Part model, mm, in its own coordinate system. A direction names the side the tool comes from. Round coordinates to 2 decimals unless told otherwise and drop trailing zeros. Write each loop counter-clockwise with the first axis right and the second up, starting at its lowest first coordinate (ties: lowest second). Pieces come first, ordered by that corner, then holes. Notation, with made-up numbers: M 41,19 L 58,19 A20 cw 58,43 Z; hole C -2.75,-4.75 d6. An arc over 180 degrees is marked long. One line per question, with ' | ' between items. Start each with the question number.
1) Saw through at C-C (z = 0). List the corners of the cut face in (x, y) (3 decimals).
2) Saw through at B-B (y = -8.75). List the corners of the cut face in (x, z) (3 decimals).
3) Saw through at A-A (x = 0). List the corners of the cut face in (y, z) (3 decimals), plus the area to 3 significant figures.
4) Drop flat-ended pins along their axis: pin 1 Ø0.5 at (x, y) = (11, -5) entering from -Z; pin 2 Ø3 at (y, z) = (-17.5, -0.5) entering from -X; pin 3 Ø4 at (y, z) = (-7.5, 5) entering from -X (3 decimals); pin 4 Ø1.5 at (x, y) = (-7, -18) entering from -Z. Give the stop position or say it passes through.
5) Saw through at D-D (y = -15.25). List the corners of the cut face in (x, z).
6) Tool access for faces 1 (the face through (-11, -5, 2.35)), 2 (the face through (-11, -5, -2.35)), 3 (the face through (10.325, -5, -5)): list every direction of +Z, -Z, +X, -X, +Y, -Y with a clear straight run to the whole face (end or side of a thin tool).
7) Wall check: probe 1 along Y at (x, z) = (11.75, 2); probe 2 along X at (y, z) = (-1.5, -5.75) (3 decimals); probe 3 along Y at (x, z) = (-2.5, 6.25). Give the ranges that are in metal, low to high. Write a range as [from, to].
```python
from build123d import *

# Parameters (mm, degrees)
F1_DEPTH = 10.2
F2_R     = 2
F3_R     = 7.65
F4_DEPTH = 6.8
F5_SIZE  = 3
F6_R     = 5.9
F7_DEPTH = 5


with BuildPart() as f1:
    # F0 (on Front) → F1 (new body)
    with BuildSketch(Plane.XZ):
        Polygon((10.325, 2.35), (10.325, 10.375), (-10.325, 10.375), (-10.325, 2.35), (-13.325, 2.35), (-13.325, -2.35), (-10.325, -2.35), (-10.325, -10.375), (10.325, -10.375), (10.325, -2.35), (13.325, -2.35), (13.325, 2.35), align=None)
    extrude(amount=F1_DEPTH)

    # F2
    f2_edges = [f1.edges().sort_by_distance(p)[0] for p in [
        (-13.325, -5.1, -2.35),
        (-13.325, -5.1, 2.35),
        (13.325, -5.1, -2.35),
        (13.325, -5.1, 2.35),
    ]]
    fillet(f2_edges, radius=F2_R)

    # F3 (on face) → F4 (join)
    with BuildSketch(Plane.XZ.offset(10.2)):
        Circle(F3_R)
    extrude(amount=F4_DEPTH)

    # F5
    f5_edges = [f1.edges().sort_by_distance(p)[0] for p in [
        (-10.325, -5.1, -10.375),
        (-10.325, -5.1, 10.375),
        (10.325, -5.1, -10.375),
        (10.325, -5.1, 10.375),
    ]]
    chamfer(f5_edges, length=F5_SIZE)

    # F6 (on face) → F7 (join)
    with BuildSketch(Plane.XZ.offset(17)):
        Circle(F6_R)
    extrude(amount=F7_DEPTH)


solid = f1.part
```
Answer key:
1) outline: M -13.325,-10.2 L -7.65,-10.2 L -7.65,-17 L -5.9,-17 L -5.9,-22 L 5.9,-22 L 5.9,-17 L 7.65,-17 L 7.65,-10.2 L 13.325,-10.2 L 13.325,0 L -13.325,0 Z
2) outline: M -13.325,-0.35 A2 ccw -11.325,-2.35 L -10.325,-2.35 L -10.325,-7.375 L -7.325,-10.375 L 7.325,-10.375 L 10.325,-7.375 L 10.325,-2.35 L 11.325,-2.35 A2 ccw 13.325,-0.35 L 13.325,0.35 A2 ccw 11.325,2.35 L 10.325,2.35 L 10.325,7.375 L 7.325,10.375 L -7.325,10.375 L -10.325,7.375 L -10.325,2.35 L -11.325,2.35 A2 ccw -13.325,0.35 Z
3) outline: M -22,-5.9 L -17,-5.9 L -17,-7.65 L -10.2,-7.65 L -10.2,-10.375 L 0,-10.375 L 0,10.375 L -10.2,10.375 L -10.2,7.65 L -17,7.65 L -17,5.9 L -22,5.9 Z | area: 375 mm2
4) pin 1: stops at z = -2.35 | pin 2: stops at x = -7.65 | pin 3: stops at x = -10.325 | pin 4: passes through
5) outline: C 0,0 d15.3
6) face 1: +Z, -X, +Y, -Y | face 2: -Z, -X, +Y, -Y | face 3: -Z, +X, +Y, -Y
7) probe 1: y = [-10.2, 0] | probe 2: x = [-10.325, 10.325] | probe 3: y = [-17, 0]
